```python
from build123d import *

# Parameters (mm, degrees)
F1_DEPTH = 3.81
F2_R     = 3.175
F3_DEPTH = 25.4


with BuildPart() as f1:
    # F0 (on Front) → F1 (new body)
    with BuildSketch(Plane.XZ):
        with BuildLine():
            Line((51.703557, 0), (-75.296443, 0))
            ThreePointArc((-75.296443, 0), (-81.646443, -6.35), (-75.296443, -12.7))
            Line((-75.296443, -12.7), (51.703557, -12.7))
            ThreePointArc((51.703557, -12.7), (58.053557, -6.35), (51.703557, 0))
        make_face()
    extrude(amount=F1_DEPTH)

    # F2 (on face) → F3 (cut)
    with BuildSketch(Plane.XZ.offset(3.81)):
        with Locations((-75.296443, -6.35)):
            Circle(F2_R)
        with Locations((0.903557, -6.35)):
            Circle(F2_R)
    extrude(amount=-F3_DEPTH, mode=Mode.SUBTRACT)


solid = f1.part
```
For this review, take the finished solid that the model builds, in its own axes (mm). Coordinates: 2 decimals unless noted, no trailing zeros. Loops run counter-clockwise (first coordinate to the right, second up) from the corner with the lowest first, then second, coordinate; pieces in that order, holes last. Notation, with made-up numbers: (-8, 7) -> (30, 7) arc R12 ccw to (30, 28) -> close; hole circle Ø4 at (18, 40.5). An arc over 180 degrees is marked (long way). Return JSON: item names as keys, results as strings. Group by question number.
(1) Mouldability with a two-part tool opening along Z and no side actions: class faces 1 (the cylindrical face through (0.22, -1.93, -9.45)), 2 (the flat face through (-13, -2, -12.7)), 3 (the cylindrical face through (-81.645, -1.878, -6.21)), 4 (the cylindrical face through (-72.268, -1.932, -5.396)) as pulls with the +Z half, pulls with the -Z half, needs draft (parallel to the pull), parting line crosses it, or undercut.
(2) To check wall thickness, follow L1, parallel to X at y = -3.05, z = -6; L2, parallel to X at y = -2.55, z = -4.25; L3, parallel to Z at x = -72.5, y = -1.1. State the ranges of each line that lie inside material, in increasing order.
(3) For pin 1 Ø1 at (y, z) = (-3, -2) entering from -X; pin 2 Ø4 at (x, z) = (0.9, -6.35) entering from -Y; pin 3 Ø1 at (y, z) = (-2.5, -7.5) entering from +X; pin 4 Ø1 at (y, z) = (-2.5, -3.5) entering from -X, all flat-tipped, find the tip position at first contact; note any pin that passes through.
(4) Consider section A-A, the plane z = -6.35. Give the boundary of the cut face in (x, y), plus the area to 3 significant figures.
(5) Consider section C-C, the plane y = -1.25. Give the boundary of the cut face in (x, z) (3 decimals), plus the area to 3 significant figures.
(6) Consider section B-B, the plane x = -0.5. Give the boundary of the cut face in (y, z).
Results below:
{
 "1": {"face 1": "undercut", "face 2": "pulls with the -Z half", "face 3": "parting line crosses it", "face 4": "undercut"},
 "2": {"L1": "x = -81.64 to -78.45, -72.14 to -2.25, 4.06 to 58.04", "L2": "x = -81.29 to -77.68, -72.92 to -1.48, 3.28 to 57.7", "L3": "z = -12.7 to -7.85, -4.85 to 0"},
 "3": {"pin 1": "stops at x = -80.35", "pin 2": "passes through", "pin 3": "stops at x = 58.02", "pin 4": "stops at x = -81.2"},
 "4": {"outline": "(-81.65, -3.81) -> (-78.47, -3.81) -> (-78.47, 0) -> (-81.65, 0) -> close; (-72.12, -3.81) -> (-2.27, -3.81) -> (-2.27, 0) -> (-72.12, 0) -> close; (4.08, -3.81) -> (58.05, -3.81) -> (58.05, 0) -> (4.08, 0) -> close", "area": "484 mm2"},
 "5": {"outline": "(-75.296, -12.7) -> (51.704, -12.7) arc R6.35 ccw to (51.704, 0) -> (-75.296, 0) arc R6.35 ccw to start; hole circle Ø6.35 at (-75.296, -6.35); hole circle Ø6.35 at (0.904, -6.35)", "area": "1,680 mm2"},
 "6": {"outline": "(-3.81, -12.7) -> (0, -12.7) -> (0, -9.2) -> (-3.81, -9.2) -> close; (-3.81, -3.5) -> (0, -3.5) -> (0, 0) -> (-3.81, 0) -> close"}
}
